The drawing under review shows one solid part. Ordinate dimensions are in mm from its lowest x, y, z. A direction names the side the tool comes from. Give positions to 0.01 mm unless a question says otherwise; leave off trailing zeros. Order: outer loops, then holes, each group sorted by start corner. A loop starts at its lowest first (then second) coordinate and runs counter-clockwise, first axis right, second up. Notation, with made-up numbers: (31.5, 41.5) - (71.5, 41.5) arc R19 ccw to (71.5, 45.5) - close; hole circle Ø9 at (36.25, 31.25). An arc over 180 degrees is marked (long way). Write item = value, one per line. Start each with the question number.
1. We need section A-A, the plane x = 30. Give the boundary of the cut face in (y, z).
2. We need section D-D, the plane z = 8. Give the boundary of the cut face in (x, y), and give its area (3 significant figures).
3. Wall thickness on probe 1 along Y at (x, z) = (4, 4.5); probe 2 along Z at (x, y) = (32, 65) (1 decimal); probe 3 along X at (y, z) = (11.5, 29): over which ranges is each line inside the solid? List them lowest first.
4. For P1, Ø5, axis at x = 32, z = 50, coming from the +Y side; P2, Ø3, axis at x = 17, y = 7.5, coming from the -Z side, all flat-tipped, find the tip position at first contact; note any pin that passes through.
5. We need section B-B, the plane z = 30. Give the boundary of the cut face in (x, y), and give its area (4 significant figures).
6. We need section C-C, the plane y = 66. Give the boundary of the cut face in (x, z), and give its area (3 significant figures).
7. Machinability: for the marked faces 1, 2 and 3, which of the approach directions +Z, -Z, +X, -X, +Y, -Y give a long, thin tool a straight path to every point of the face, cutting with its end or side? Answer none if there is none.
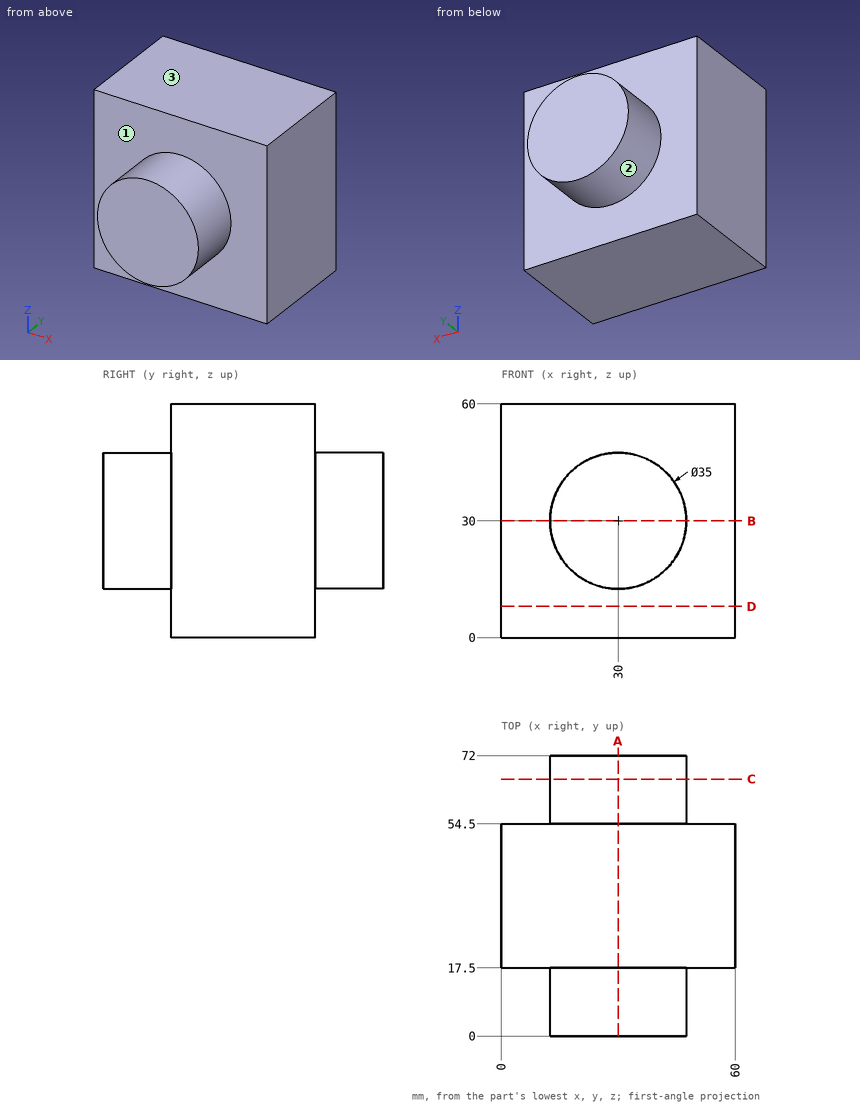
Model answer:
q1.outline = (0, 12.5) - (17.5, 12.5) - (17.5, 0) - (54.5, 0) - (54.5, 12.5) - (72, 12.5) - (72, 47.5) - (54.5, 47.5) - (54.5, 60) - (17.5, 60) - (17.5, 47.5) - (0, 47.5) - close
q2.outline = (0, 17.5) - (60, 17.5) - (60, 54.5) - (0, 54.5) - close
q2.area = 2,220 mm2
q3.probe_1 = 17.5 to 54.5
q3.probe_2 = 12.6 to 47.4
q3.probe_3 = 12.53 to 47.47
q4.P1 = 54.5
q4.P2 = 16.81
q5.outline = (0, 17.5) - (12.5, 17.5) - (12.5, 0) - (47.5, 0) - (47.5, 17.5) - (60, 17.5) - (60, 54.5) - (47.5, 54.5) - (47.5, 72) - (12.5, 72) - (12.5, 54.5) - (0, 54.5) - close
q5.area = 3,445 mm2
q6.outline = circle Ø35 at (30, 30)
q6.area = 962 mm2
q7.face_1 = -Y
q7.face_2 = +Y
q7.face_3 = +Z, +X, -X, +Y, -Y
